Job drawing, mm, ordinate dimensions from the low corner. One solid piece. A direction names the side the tool comes from. Round coordinates to 2 decimals unless told otherwise and drop trailing zeros. Loops run counter-clockwise (first coordinate to the right, second up) from the corner with the lowest first, then second, coordinate; pieces in that order, holes last. Notation, with made-up numbers: M -7,5 L 41,5 A31 cw 41,42 Z; hole C 56.5,16 d5. An arc over 180 degrees is marked long. Use one line per item in the form item = value.
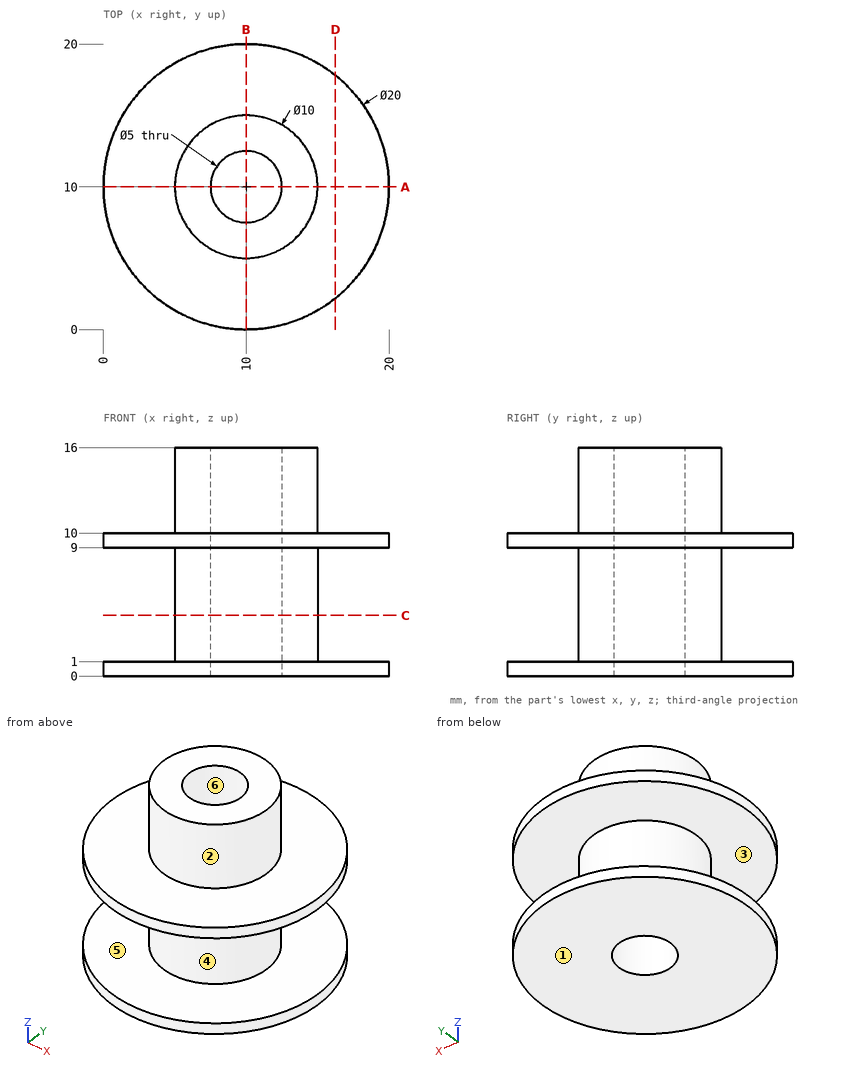
1. Cut at D-D on x = 16.25. Write the cut outline in (y, z), and give its area (3 significant figures).
Completed:
outline = M 2.19,0 L 17.81,0 L 17.81,1 L 2.19,1 Z; M 2.19,9 L 17.81,9 L 17.81,10 L 2.19,10 Z
area = 31.2 mm2
2. Drop flat-ended pins along their axis: P1, Ø12, axis at x = 6.5, y = 5, coming from the -Z side; P2, Ø1, axis at x = 6.5, z = 9, coming from the +Y side; P3, Ø1.5, axis at x = 9, z = 3, coming from the +Y side; P4, Ø1.5, axis at x = 4.5, z = 8.5, coming from the -Y side. Give the stop position or say it passes through.
Completed:
P1 = 0
P2 = 19.54
P3 = 14.99
P4 = 1.31
3. Pull direction X, two halves, no side cores. Call the marked faces 4, 5 and 6: +X half, -X half, draft (parallel to the pull), parting line (faces both ways), or undercut.
Completed:
face_4 = parting line
face_5 = draft
face_6 = undercut
4. Tool access for the marked faces 1, 2 and 3: list every direction of +Z, -Z, +X, -X, +Y, -Y with a clear straight run to the whole face (end or side of a thin tool).
Completed:
face_1 = -Z, +X, -X, +Y, -Y
face_2 = +Z
face_3 = none
5. Probe line 1 along Y through (x, z) = (10, 8.75); line 2 along Z through (x, y) = (4.5, 8.25); line 3 along Y through (x, z) = (10.5, 3.75). List the from-to ranges inside material, lowest first. Write a range as from..to.
Completed:
line_1 = 5..7.5, 12.5..15
line_2 = 0..1, 9..10
line_3 = 5.03..7.55, 12.45..14.97
6. Cut at C-C on z = 4.25. Write the cut outline in (x, y), and give its area (3 significant figures).
Completed:
outline = C 10,10 d10; hole C 10,10 d5
area = 58.9 mm2
7. Cut at A-A on y = 10. Write the cut outline in (x, z).
Completed:
outline = M 0,0 L 7.5,0 L 7.5,16 L 5,16 L 5,10 L 0,10 L 0,9 L 5,9 L 5,1 L 0,1 Z; M 12.5,0 L 20,0 L 20,1 L 15,1 L 15,9 L 20,9 L 20,10 L 15,10 L 15,16 L 12.5,16 Z
